Can you work these out from the model? Positions are in its coordinate system, mm. Give positions to 0.01 mm unless a question says otherwise; leave off trailing zeros. Loops run counter-clockwise (first coordinate to the right, second up) from the corner with the lowest first, then second, coordinate; pieces in that order, holes last.
from build123d import *

# Parameters (mm, degrees)
F0_R     = 37.5
F0_R_2   = 27.5
F1_DEPTH = 82
F2_DEPTH = 5
F3_R     = 15
F4_R     = 5
F5_R     = 4.99999


# Not quite as in the source:
# - a fillet or chamfer is up to 0.001 mm smaller than in the source, because OpenCascade refuses the exact size


with BuildPart() as f1:
    # F0 (on Top) → F1 (new body)
    with BuildSketch(Plane.XY):
        Circle(F0_R)
        Circle(F0_R_2, mode=Mode.SUBTRACT)
    extrude(amount=F1_DEPTH)

    # F0 (on Top) → F2 (join)
    with BuildSketch(Plane.XY):
        Circle(F0_R_2)
    extrude(amount=F2_DEPTH)

    # F3
    f3_edges = [f1.edges().sort_by_distance(p)[0] for p in [
        (-37.5, 0, 0),
    ]]
    fillet(f3_edges, radius=F3_R)

    # F4
    f4_edges = [f1.edges().sort_by_distance(p)[0] for p in [
        (-37.5, 0, 82),
    ]]
    fillet(f4_edges, radius=F4_R)

    # F5 (radius 5 in the source; OpenCascade refuses exactly that, so slightly less here)
    f5_edges = [f1.edges().sort_by_distance(p)[0] for p in [
        (-27.5, 0, 82),
    ]]
    fillet(f5_edges, radius=F5_R)


solid = f1.part
(1) Thinking about a two-plate mould opening in Y: for faces 1 (the flat face through (0, 0, 5)), 2 (the cylindrical face through (-4.88, 37.18, 45.57)), 3 (the cylindrical face through (-5.961, -26.846, 40.496)), 4 (the flat face through (0, 0, 0)), which applies, pulls with the +Y half, pulls with the -Y half, needs draft (parallel to the pull), parting line crosses it, or undercut?
Returned:
face 1: undercut
face 2: parting line crosses it
face 3: undercut
face 4: needs draft
(2) Suppose I cut it at C-C on z = 17. List the corners of the cut face in (x, y) for me.
Returned:
outline: circle Ø75 at (0, 0); hole circle Ø55 at (0, 0)
(3) Please list where these lines run through material, in increasing order: probe 1 along Y at (x, z) = (0, 39); probe 2 along Z at (x, y) = (-10.5, 16.5); probe 3 along X at (y, z) = (12, 59).
Returned:
probe 1: y = -37.5 to -27.5, 27.5 to 37.5
probe 2: z = 0 to 5
probe 3: x = -35.53 to -24.74, 24.74 to 35.53
(4) Will these pins go through, and if not, where does the flat tip stop? P1, Ø1, axis at x = 6.5, z = 68, coming from the -Y side; P2, Ø6, axis at y = -21.5, z = 53, coming from the +X side; P3, Ø10, axis at x = -18.5, y = -23, coming from the +Z side; P4, Ø6, axis at x = 13, z = 56, coming from the -Y side.
Returned:
P1: stops at y = -37.02
P2: stops at x = 32.62
P3: stops at z = 82
P4: stops at y = -36.14
